```python
from build123d import *

# Parameters (mm, degrees)
F1_DEPTH = 100
F2_R     = 7.0395
F6_DEPTH = 10


with BuildPart() as f1:
    # F0 (on Top) → F1 (new body)
    with BuildSketch(Plane.XY):
        Polygon((20.710678, 50), (-20.710678, 50), (-50, 20.710678), (-50, -20.710678), (-20.710678, -50), (20.710678, -50), (50, -20.710678), (50, -9.2725), (50, 9.2725), (50, 20.710678), align=None)
        Polygon((-40, 16.568542), (-16.568542, 40), (16.568542, 40), (40, 16.568542), (40, -16.568542), (16.568542, -40), (-16.568542, -40), (-40, -16.568542), align=None, mode=Mode.SUBTRACT)
    extrude(amount=F1_DEPTH)

    # F4: sweep along a path in F3
    with BuildLine(Plane.XZ) as f4_path:
        ThreePointArc((49.790855, 24.170094), (76.688355, 51.067594), (49.790855, 77.965094))
    # F2 (on face) → F4 (sweep)
    with BuildSketch(Plane.YZ.offset(50)):
        with Locations((0, 77.352941)):
            Circle(F2_R)
    sweep(path=f4_path.line)

    # F5 (on Top) → F6 (join)
    with BuildSketch(Plane.XY):
        Polygon((-18.548241, -44.779416), (18.548241, -44.779416), (44.779416, -18.548241), (44.779416, 18.548241), (18.548241, 44.779416), (-18.548241, 44.779416), (-44.779416, 18.548241), (-44.779416, -18.548241), align=None)
    extrude(amount=-F6_DEPTH)


solid = f1.part
```
Source: CAD feature listing. Evaluate the final solid. Frame: model axes, mm. A direction names the side the tool comes from. Give positions to 0.01 mm unless a question says otherwise; leave off trailing zeros. Loops run counter-clockwise (first coordinate to the right, second up) from the corner with the lowest first, then second, coordinate; pieces in that order, holes last. Notation, with made-up numbers: (-35.5, 84.25) -> (-15.5, 84.25) arc R14 ccw to (-15.5, 88.25) -> close; hole circle Ø3 at (60, -26.75). An arc over 180 degrees is marked (long way). Use a Markdown table: item, result. Add a question column.
(1) First-contact query: pin 1 Ø5 at (x, z) = (-6.5, -6) entering from +Y; pin 2 Ø10 at (y, z) = (7.5, 60.5) entering from +X; pin 3 Ø4 at (x, y) = (-14.5, 18) entering from +Z; pin 4 Ø12 at (x, y) = (64.5, -16.5) entering from +Z. Flat tips, straight axial feed; report the tip coordinate or a pass-through.
(2) Section query C-C (z = 4.5). Output: boundary loops of the cut face in (x, y).
(3) Pull-direction query (Y, two-part tool) for faces 6 (the face through (-28.45, 28.12, 49.3)), 7 (the face through (-1, 1, -10)), 8 (the face through (-31.48, 31.85, -4.93)); classes: +Y half, -Y half, draft (parallel to the pull), parting line (faces both ways), or undercut.
(4) Section query D-D (z = 38). Count the separate pieces of the cut face and the enclosed holes in it, then the cut area to 3 significant figures.
(5) Section query A-A (y = -10). Output: boundary loops of the cut face in (x, z).
(6) Access query for faces 1 (the face through (0, -40, 49)), 2 (the face through (-44.779, 0, -5)), 3 (the face through (0, 44.779, -5)), 4 (the face through (-31.85, -31.48, -4.93)), 5 (the face through (44.779, 0, -5)). Directions: +Z, -Z, +X, -X, +Y, -Y. A direction counts if a zero-diameter tool reaches every point of the face in a straight line with its end or side. Return the directions, or none.
(7) Ray query, line 1 (X direction, y = 14, z = 77); line 2 (X direction, y = 6, z = 37); line 3 (Y direction, x = -39, z = 3). Return the intervals inside material, ascending.
Checked values:
| question | item | result |
|---|---|---|
| 1 | pin 1 | y = 44.78 |
| 1 | pin 2 | x = 81.63 |
| 1 | pin 3 | z = 0 |
| 1 | pin 4 | through |
| 2 | outline | (-50, -20.71) -> (-20.71, -50) -> (20.71, -50) -> (50, -20.71) -> (50, 20.71) -> (20.71, 50) -> (-20.71, 50) -> (-50, 20.71) -> close; hole (-40, -16.57) -> (-16.57, -40) -> (16.57, -40) -> (40, -16.57) -> (40, 16.57) -> (16.57, 40) -> (-16.57, 40) -> (-40, 16.57) -> close |
| 3 | face 6 | undercut |
| 3 | face 7 | draft |
| 3 | face 8 | +Y half |
| 4 | separate pieces | 2 |
| 4 | enclosed holes | 1 |
| 4 | area | 3,160 mm^2 |
| 5 | outline | (-50, 0) -> (-44.78, 0) -> (-44.78, -10) -> (44.78, -10) -> (44.78, 0) -> (50, 0) -> (50, 100) -> (40, 100) -> (40, 0) -> (-40, 0) -> (-40, 100) -> (-50, 100) -> close |
| 6 | face 1 | +Z |
| 6 | face 2 | -Z, -X, +Y, -Y |
| 6 | face 3 | -Z, +X, -X, +Y |
| 6 | face 4 | -Z, -X, -Y |
| 6 | face 5 | -Z, +X, +Y, -Y |
| 7 | line 1 | -50 to -40, 40 to 50 |
| 7 | line 2 | -50 to -40, 40 to 50, 67.48 to 76.25 |
| 7 | line 3 | -31.71 to -17.57, 17.57 to 31.71 |
